Can you work these out from the model? Positions are in its coordinate system, mm. A direction names the side the tool comes from. Round coordinates to 2 decimals unless told otherwise and drop trailing zeros. Loops run counter-clockwise (first coordinate to the right, second up) from the corner with the lowest first, then second, coordinate; pieces in that order, holes last.
(1) I want a section at C-C on y = 3.5. Give the number of separate pieces and of enclosed holes in the cut face, plus the area to 3 significant figures.
(2) I want a section at B-B on z = 0. Write out the boundary of the cut face in (x, y), plus the area to 3 significant figures.
(3) I want a section at D-D on y = 18. Write out the boundary of the cut face in (x, z).
(4) Thinking about a two-plate mould opening in Z: for faces 4 (the face through (-13, 0, -12)), 5 (the face through (22, 5, 13)), 6 (the face through (0, 49, 27)), which applies, released by +Z, released by -Z, zero draft, split by the parting line, or undercut?
(5) Which directions (+Z, -Z, +X, -X, +Y, -Y) give clear straight access to the entire face, cutting with the end or side of a thin tool? Please do faces 1 (the face through (-13, 47, 13)), 2 (the face through (10.916, 25.636, -26.327)), 3 (the face through (22.495, 2.465, 13.421)).
(6) If I drill on line 1 along Z through (x, y) = (-14.5, 48); line 2 along X through (y, z) = (3.4, 12.5); line 3 along X through (y, z) = (4, -13.5), over which ranges is the centre line in solid material (lowest first)?
(7) Will these pins go through, and if not, where does the flat tip stop? pin 1 Ø8 at (y, z) = (4.5, -15) entering from +X; pin 2 Ø0.8 at (x, z) = (13, -13.5) entering from +Y; pin 3 Ø3 at (x, z) = (-21.5, 13) entering from -Y.
from build123d import *

# Parameters (mm, degrees)
SKETCH_1_R          = 28.5
EXTRUDE_1_DEPTH     = 52
SKETCH_2_R          = 17.5
EXTRUDE_2_DEPTH     = 1
SKETCH_3_R          = 1.25
SKETCH_3_R_2        = 4.75
CUT_EXTRUDE_1_DEPTH = 3.5
MOVE_FACE_1_BY      = 3.5
MOVE_FACE_1_2_BY    = 3.5
MOVE_FACE_1_3_BY    = 3.5
MOVE_FACE_1_4_BY    = 3.5
MOVE_FACE_1_5_BY    = 3.5
MOVE_FACE_1_6_BY    = 3.5
SKETCH_4_R          = 1.25
CUT_EXTRUDE_2_DEPTH = 5
SKETCH_5_W          = 15.5
SKETCH_5_H          = 4.5
CUT_EXTRUDE_3_DEPTH = 1.5
SKETCH_6_R          = 1.25
CUT_EXTRUDE_4_DEPTH = 5


with BuildPart() as part:
    # Sketch 1 → Extrude 1 (new body)
    with BuildSketch(Plane(origin=(0, 0, 0), x_dir=(1, 0, 0), z_dir=(0, 1, 0))):
        with Locations(Location((0, 0, 0), (0, 0, 90))):
            Circle(SKETCH_1_R)
    extrude(amount=EXTRUDE_1_DEPTH)

    # Sketch 2 → Extrude 2 (add)
    with BuildSketch(Plane.XZ):
        with Locations(Location((0, 0, 0), (0, 0, 270))):
            Circle(SKETCH_2_R)
    extrude(amount=EXTRUDE_2_DEPTH)

    # Sketch 3 → Cut-Extrude 1 (cut)
    with BuildSketch(Plane.XZ.offset(1)):
        with Locations(Location((0, 13.5, 0), (0, 0, 270))):
            Circle(SKETCH_3_R)
        with Locations(Location((11.691342951, 6.75, 0), (0, 0, 270))):
            Circle(SKETCH_3_R)
        with Locations(Location((11.691342951, -6.75, 0), (0, 0, 270))):
            Circle(SKETCH_3_R)
        with Locations(Location((0, -13.5, 0), (0, 0, 270))):
            Circle(SKETCH_3_R)
        with Locations(Location((-11.691342951, -6.75, 0), (0, 0, 270))):
            Circle(SKETCH_3_R)
        with Locations(Location((-11.691342951, 6.75, 0), (0, 0, 270))):
            Circle(SKETCH_3_R)
        with Locations(Location((0, 0, 0), (0, 0, 270))):
            Circle(SKETCH_3_R_2)
    extrude(amount=-CUT_EXTRUDE_1_DEPTH, mode=Mode.SUBTRACT)

    # Move Face 1: a face moved inward by 3.5
    extrude(part.faces().sort_by_distance((11.691342951, 2.5, -6.75))[0], amount=MOVE_FACE_1_BY, dir=(0, 1, 0), mode=Mode.SUBTRACT)

    # Move Face 1 2: a face moved inward by 3.5
    extrude(part.faces().sort_by_distance((0, 2.5, -13.5))[0], amount=MOVE_FACE_1_2_BY, dir=(0, 1, 0), mode=Mode.SUBTRACT)

    # Move Face 1 3: a face moved inward by 3.5
    extrude(part.faces().sort_by_distance((-11.691342951, 2.5, -6.75))[0], amount=MOVE_FACE_1_3_BY, dir=(0, 1, 0), mode=Mode.SUBTRACT)

    # Move Face 1 4: a face moved inward by 3.5
    extrude(part.faces().sort_by_distance((-11.691342951, 2.5, 6.75))[0], amount=MOVE_FACE_1_4_BY, dir=(0, 1, 0), mode=Mode.SUBTRACT)

    # Move Face 1 5: a face moved inward by 3.5
    extrude(part.faces().sort_by_distance((0, 2.5, 13.5))[0], amount=MOVE_FACE_1_5_BY, dir=(0, 1, 0), mode=Mode.SUBTRACT)

    # Move Face 1 6: a face moved inward by 3.5
    extrude(part.faces().sort_by_distance((11.691342951, 2.5, 6.75))[0], amount=MOVE_FACE_1_6_BY, dir=(0, 1, 0), mode=Mode.SUBTRACT)

    # Sketch 4 → Cut-Extrude 2 (cut)
    with BuildSketch(Plane.XZ):
        with Locations(Location((0, 25, 0), (0, 0, 270))):
            Circle(SKETCH_4_R)
        with Locations(Location((21.650635095, 12.5, 0), (0, 0, 270))):
            Circle(SKETCH_4_R)
        with Locations(Location((21.650635095, -12.5, 0), (0, 0, 270))):
            Circle(SKETCH_4_R)
        with Locations(Location((0, -25, 0), (0, 0, 270))):
            Circle(SKETCH_4_R)
        with Locations(Location((-21.650635095, -12.5, 0), (0, 0, 270))):
            Circle(SKETCH_4_R)
        with Locations(Location((-21.650635095, 12.5, 0), (0, 0, 270))):
            Circle(SKETCH_4_R)
    extrude(amount=-CUT_EXTRUDE_2_DEPTH, mode=Mode.SUBTRACT)

    # Sketch 5 → Cut-Extrude 3 (cut)
    with BuildSketch(Plane.XY.offset(28.5)):
        with Locations((0, 48.75)):
            Rectangle(SKETCH_5_W, SKETCH_5_H)
    extrude(amount=-CUT_EXTRUDE_3_DEPTH, mode=Mode.SUBTRACT)

    # Sketch 6 → Cut-Extrude 4 (cut)
    with BuildSketch(Plane(origin=(0, 52, 0), x_dir=(1, 0, 0), z_dir=(0, 1, 0))):
        with Locations(Location((13.435028843, 13.435028843, 0), (0, 0, 270))):
            Circle(SKETCH_6_R)
        with Locations(Location((13.435028843, -13.435028843, 0), (0, 0, 270))):
            Circle(SKETCH_6_R)
        with Locations(Location((-13.435028843, -13.435028843, 0), (0, 0, 270))):
            Circle(SKETCH_6_R)
        with Locations(Location((-13.435028843, 13.435028843, 0), (0, 0, 270))):
            Circle(SKETCH_6_R)
    extrude(amount=-CUT_EXTRUDE_4_DEPTH, mode=Mode.SUBTRACT)


solid = part.part
Filled sheet:
1. separate pieces: 1
1. enclosed holes: 12
1. area: 2,490 mm2
2. outline: (-28.5, 0) - (-17.5, 0) - (-17.5, -1) - (-4.75, -1) - (-4.75, 2.5) - (4.75, 2.5) - (4.75, -1) - (17.5, -1) - (17.5, 0) - (28.5, 0) - (28.5, 52) - (-28.5, 52) - close
2. area: 2,970 mm2
3. outline: circle Ø57 at (0, 0)
4. face 4: zero draft
4. face 5: undercut
4. face 6: released by +Z
5. face 1: +Y
5. face 2: +Y, -Y
5. face 3: -Y
6. line 1: z = -24.54 to -14.09, -12.78 to 12.78, 14.09 to 24.54
6. line 2: x = -25.61 to -22.9, -20.4 to -0.75, 0.75 to 20.4, 22.9 to 25.61
6. line 3: x = -25.1 to -22.4, -20.9 to -1.25, 1.25 to 20.9, 22.4 to 25.1
7. pin 1: stops at x = 26.29
7. pin 2: stops at y = 47
7. pin 3: stops at y = 0
